from build123d import *

# Parameters (mm, degrees)
SKETCH2_W           = 101.6
SKETCH2_H           = 50.8
BOSS_EXTRUDE1_DEPTH = 8
SKETCH3_W           = 51
SKETCH3_H           = 16
CUT_EXTRUDE1_DEPTH  = 58.356778152
FILLET1_R           = 8
SKETCH5_R           = 1.63195
CUT_EXTRUDE2_DEPTH  = 58.356778152
SKETCH6_R           = 1.63195
CUT_EXTRUDE3_DEPTH  = 58.356778152
SKETCH7_W           = 10.16
SKETCH7_H           = 6.016
CUT_EXTRUDE4_DEPTH  = 58.356778152
SKETCH8_W           = 10.16
SKETCH8_H           = 6.016
CUT_EXTRUDE5_DEPTH  = 58.356778152
SKETCH9_R           = 2.794
CUT_EXTRUDE6_DEPTH  = 2.032
SKETCH10_R          = 2.794
CUT_EXTRUDE7_DEPTH  = 2.032


with BuildPart() as part:
    # Sketch2 → Boss-Extrude1 (new body)
    with BuildSketch(Plane(origin=(0, 0, 0), x_dir=(1, 0, 0), z_dir=(0, 1, 0))):
        Rectangle(SKETCH2_W, SKETCH2_H)
    extrude(amount=BOSS_EXTRUDE1_DEPTH)

    # Sketch3 → Cut-Extrude1 (cut, through all)
    with BuildSketch(Plane(origin=(0, 8, 0), x_dir=(1, 0, 0), z_dir=(0, 1, 0))):
        Rectangle(SKETCH3_W, SKETCH3_H)
    extrude(amount=-CUT_EXTRUDE1_DEPTH, mode=Mode.SUBTRACT)

    # Fillet1
    fillet1_edges = [part.edges().sort_by_distance(p)[0] for p in [
        (0, 8, -25.4),
        (50.8, 8, 0),
        (0, 8, 25.4),
        (-50.8, 8, 0),
    ]]
    fillet(fillet1_edges, radius=FILLET1_R - 0.0001)  # a hair under: the kernel refuses the full size

    # Sketch5 → Cut-Extrude2 (cut, through all)
    with BuildSketch(Plane.XZ):
        with Locations(Location((-33.1, 0, 0), (0, 0, 270))):
            Circle(SKETCH5_R)
    extrude(amount=-CUT_EXTRUDE2_DEPTH, mode=Mode.SUBTRACT)

    # Sketch6 → Cut-Extrude3 (cut, through all)
    with BuildSketch(Plane.XZ):
        with Locations(Location((33.1, 0, 0), (0, 0, 270))):
            Circle(SKETCH6_R)
    extrude(amount=-CUT_EXTRUDE3_DEPTH, mode=Mode.SUBTRACT)

    # Sketch7 → Cut-Extrude4 (cut, through all)
    with BuildSketch(Plane.XZ):
        with Locations((0, 22.392)):
            Rectangle(SKETCH7_W, SKETCH7_H)
    extrude(amount=-CUT_EXTRUDE4_DEPTH, mode=Mode.SUBTRACT)

    # Sketch8 → Cut-Extrude5 (cut, through all)
    with BuildSketch(Plane.XZ):
        with Locations((0, -22.392)):
            Rectangle(SKETCH8_W, SKETCH8_H)
    extrude(amount=-CUT_EXTRUDE5_DEPTH, mode=Mode.SUBTRACT)

    # Sketch9 → Cut-Extrude6 (cut)
    with BuildSketch(Plane(origin=(0, 8, 0), x_dir=(1, 0, 0), z_dir=(0, 1, 0))):
        with Locations(Location((-33.1, 0, 0), (0, 0, 270))):
            Circle(SKETCH9_R)
    extrude(amount=-CUT_EXTRUDE6_DEPTH, mode=Mode.SUBTRACT)

    # Sketch10 → Cut-Extrude7 (cut)
    with BuildSketch(Plane(origin=(0, 8, 0), x_dir=(1, 0, 0), z_dir=(0, 1, 0))):
        with Locations(Location((33.1, 0, 0), (0, 0, 270))):
            Circle(SKETCH10_R)
    extrude(amount=-CUT_EXTRUDE7_DEPTH, mode=Mode.SUBTRACT)


solid = part.part
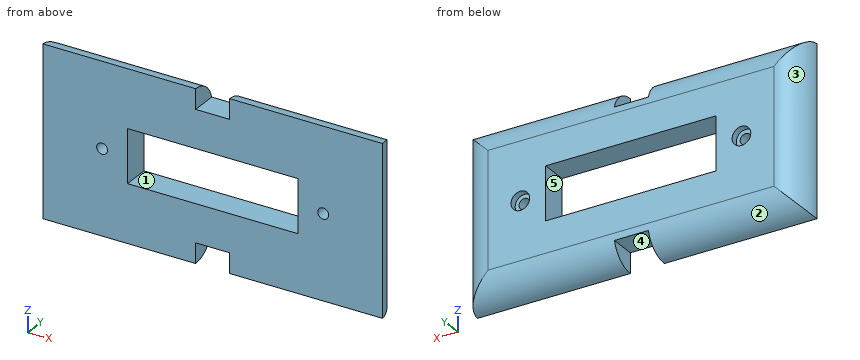
Can you work these out from the model? Positions are in its coordinate system, mm. Face numbers are marked on the shaded views. A direction names the side the tool comes from. Give positions to 0.01 mm unless a question says otherwise; leave off trailing zeros. Answer as a JSON object with one key per item and string values. Group by question number.
Item 1: I'm going to push flat-ended pins straight in: P1, Ø2, axis at y = 4.5, z = -10.5, coming from the +X side; P2, Ø4, axis at x = 10, y = 5.5, coming from the +Z side; P3, Ø1.8, axis at y = 2.5, z = 22.5, coming from the +X side. Where does each tip first touch, or does it pass through?
Item 2: Suppose I cut it at C-C (z = 0). State how many separate pieces and enclosed holes the cut face has, plus the area to 3 significant figures.
Item 3: We'd pull the mould along Z, two halves only. Please class the marked faces 3, 4 and 5: +Z half, -Z half, draft (parallel to the pull), parting line (faces both ways), or undercut.
Item 4: For the marked faces 1 and 2, which set-ups out of +Z, -Z, +X, -X, +Y, -Y let a thin tool reach every point of the face, with its end or its side?
Item 5: Please list where these lines run through material, in increasing order: line 1 (X direction, y = 1.6, z = 0); line 2 (X direction, y = 6.4, z = 0); line 3 (Z direction, x = 4.5, y = 3.75). Write a range as [from, to].
Findings:
{
 "1": {"P1": "stops at x = 49.99", "P2": "stops at z = 24.59", "P3": "stops at x = 50.64"},
 "2": {"separate pieces": "4", "enclosed holes": "0", "area": "316 mm²"},
 "3": {"face 3": "draft", "face 4": "-Z half", "face 5": "undercut"},
 "4": {"face 1": "+Y, -Y", "face 2": "-Z, +X, -X, +Y"},
 "5": {"line 1": "x = [-50.64, -34.73], [-31.47, -25.5], [25.5, 31.47], [34.73, 50.64]", "line 2": "x = [-47.6, -35.89], [-30.31, -25.5], [25.5, 30.31], [35.89, 47.6]", "line 3": "z = [-19.38, -8], [8, 19.38]"}
}
